Design review of the part built by this model. Coordinates are the model's own, in mm. Give positions to 0.01 mm unless a question says otherwise; leave off trailing zeros. Write each loop counter-clockwise with the first axis right and the second up, starting at its lowest first coordinate (ties: lowest second). Pieces come first, ordered by that corner, then holes. Notation, with made-up numbers: M -23,-39 L 12,-39 A6 cw 12,-34 Z; hole C 37.25,-20.75 d4. An arc over 180 degrees is marked long. Answer in a Markdown table with one row per item.
```python
from build123d import *

# Parameters (mm, degrees)
SKETCH1_W               = 105
SKETCH1_H               = 192.3454
BOSS_EXTRUDE1_DEPTH     = 3.175
CHAMFER1_SIZE           = 3.5
SKETCH2_R               = 25
CUT_EXTRUDE1_DEPTH      = 110.615322151
CUT_EXTRUDE_THIN1_START = -1
CUT_EXTRUDE_THIN1_DEPTH = 1
CUT_EXTRUDE2_DEPTH      = 1
SKETCH6_R               = 1.1
CUT_EXTRUDE3_DEPTH      = 110.615322151
CHAMFER2_SIZE           = 1.1


# Read off the part's stored shape, not the designer's step: Cut-Extrude-Thin1
with BuildPart() as part:
    # Sketch1 → Boss-Extrude1 (new body)
    with BuildSketch(Plane(origin=(0, 0, 0), x_dir=(1, 0, 0), z_dir=(0, 1, 0))):
        Rectangle(SKETCH1_W, SKETCH1_H)
    extrude(amount=BOSS_EXTRUDE1_DEPTH)

    # Chamfer1
    chamfer1_edges = [part.edges().sort_by_distance(p)[0] for p in [
        (-52.5, 1.5875, -96.1727),
        (52.5, 1.5875, -96.1727),
        (52.5, 1.5875, 96.1727),
        (-52.5, 1.5875, 96.1727),
    ]]
    chamfer(chamfer1_edges, length=CHAMFER1_SIZE)

    # Sketch2 → Cut-Extrude1 (cut, through all)
    with BuildSketch(Plane.XZ):
        with Locations(Location((0, -32.057566667, 0), (0, 0, 270))):
            Circle(SKETCH2_R)
    extrude(amount=-CUT_EXTRUDE1_DEPTH, mode=Mode.SUBTRACT)

    # Cut-Extrude-Thin1 outline → Cut-Extrude-Thin1 (cut)
    # profile 1 of 2: a face of its own
    with BuildSketch(Plane(origin=(0, 0, 0), x_dir=(-1, 0, 0), z_dir=(0, -1, 0)).offset(CUT_EXTRUDE_THIN1_START)):
        with BuildLine():
            Line((-0.5, 7.062567167), (-0.5, -10.4787141))
            ThreePointArc((-0.5, -10.4787141), (-6.237149669, -19.303333464), (-7.980739941, -29.683539926))
            ThreePointArc((-7.980739941, -29.683539926), (0, -26.804235846), (7.980739941, -29.683539926))
            ThreePointArc((7.980739941, -29.683539926), (6.237149669, -19.303333464), (0.5, -10.4787141))
            Line((0.5, -10.4787141), (0.5, 7.062567167))
            ThreePointArc((0.5, 7.062567167), (0, 7.057566667), (-0.5, 7.062567167))
        make_face()
        with BuildLine():
            ThreePointArc((0, -11.397130906), (5.003923805, -18.927747814), (6.982377972, -27.750171719))
            ThreePointArc((6.982377972, -27.750171719), (0, -25.804235846), (-6.982377972, -27.750171719))
            ThreePointArc((-6.982377972, -27.750171719), (-5.003923805, -18.927747814), (0, -11.397130906))
        make_face(mode=Mode.SUBTRACT)
    # profile 2 of 2: a face of its own
    with BuildSketch(Plane(origin=(0, 0, 0), x_dir=(-1, 0, 0), z_dir=(0, -1, 0)).offset(CUT_EXTRUDE_THIN1_START)):
        with BuildLine():
            ThreePointArc((-3.461538462, -73.83767702), (-2.032623324, -72.965633547), (-0.5, -72.292340123))
            Line((-0.5, -72.292340123), (-0.5, -96.1727))
            Line((-0.5, -96.1727), (0.5, -96.1727))
            Line((0.5, -96.1727), (0.5, -89.050988889))
            Line((0.5, -89.050988889), (5.5, -89.050988889))
            Line((5.5, -89.050988889), (5.5, -88.050988889))
            Line((5.5, -88.050988889), (0.5, -88.050988889))
            Line((0.5, -88.050988889), (0.5, -71.977550364))
            ThreePointArc((0.5, -71.977550364), (3.75, -71.547658069), (7, -71.977550364))
            Line((7, -71.977550364), (7, -96.1727))
            Line((7, -96.1727), (8, -96.1727))
            Line((8, -96.1727), (8, -81.550988889))
            Line((8, -81.550988889), (32.5, -81.550988889))
            Line((32.5, -81.550988889), (32.5, 13.3273))
            Line((32.5, 13.3273), (39, 13.3273))
            Line((39, 13.3273), (39, -88.050988889))
            Line((39, -88.050988889), (9.5, -88.050988889))
            Line((9.5, -88.050988889), (9.5, -89.050988889))
            Line((9.5, -89.050988889), (40, -89.050988889))
            Line((40, -89.050988889), (40, 13.3273))
            Line((40, 13.3273), (43.75, 13.3273))
            Line((43.75, 13.3273), (43.75, 24.3273))
            ThreePointArc((43.75, 24.3273), (41.580951895, 29.804525575), (36.25, 32.311659711))
            Line((36.25, 32.311659711), (36.25, 63.444142327))
            Line((36.25, 63.444142327), (4.25, 63.444142327))
            Line((4.25, 63.444142327), (4.25, 68.752070988))
            ThreePointArc((4.25, 68.752070988), (6.207809813, 67.846319731), (7.980739941, 66.617448963))
            ThreePointArc((7.980739941, 66.617448963), (6.237149669, 76.997655425), (0.5, 85.822274789))
            Line((0.5, 85.822274789), (0.5, 96.1727))
            Line((0.5, 96.1727), (-0.5, 96.1727))
            Line((-0.5, 96.1727), (-0.5, 85.822274789))
            ThreePointArc((-0.5, 85.822274789), (-6.237149669, 76.997655425), (-7.980739941, 66.617448963))
            ThreePointArc((-7.980739941, 66.617448963), (-6.207809813, 67.846319731), (-4.25, 68.752070988))
            Line((-4.25, 68.752070988), (-4.25, 63.444142327))
            Line((-4.25, 63.444142327), (-36.25, 63.444142327))
            Line((-36.25, 63.444142327), (-36.25, 32.311659711))
            ThreePointArc((-36.25, 32.311659711), (-41.580951895, 29.804525575), (-43.75, 24.3273))
            Line((-43.75, 24.3273), (-43.75, 13.3273))
            Line((-43.75, 13.3273), (-40, 13.3273))
            Line((-40, 13.3273), (-40, -96.1727))
            Line((-40, -96.1727), (-39, -96.1727))
            Line((-39, -96.1727), (-39, -38.185855556))
            Line((-39, -38.185855556), (-3.25, -38.185855556))
            Line((-3.25, -38.185855556), (-3.25, -29.234128142))
            ThreePointArc((-3.25, -29.234128142), (0, -28.804235846), (3.25, -29.234128142))
            Line((3.25, -29.234128142), (3.25, -44.685855556))
            Line((3.25, -44.685855556), (-31.5, -44.685855556))
            Line((-31.5, -44.685855556), (-31.5, -39.685855556))
            Line((-31.5, -39.685855556), (-32.5, -39.685855556))
            Line((-32.5, -39.685855556), (-32.5, -45.685855556))
            Line((-32.5, -45.685855556), (3.25, -45.685855556))
            Line((3.25, -45.685855556), (3.25, -53.222136322))
            ThreePointArc((3.25, -53.222136322), (-2.487149669, -62.046755686), (-4.230739941, -72.426962148))
            ThreePointArc((-4.230739941, -72.426962148), (3.75, -69.547658069), (11.730739941, -72.426962148))
            ThreePointArc((11.730739941, -72.426962148), (9.987149669, -62.046755686), (4.25, -53.222136322))
            Line((4.25, -53.222136322), (4.25, -29.548917901))
            ThreePointArc((4.25, -29.548917901), (5.782623324, -30.222211325), (7.211538462, -31.094254798))
            Line((7.211538462, -31.094254798), (7.788461538, -30.277456314))
            ThreePointArc((7.788461538, -30.277456314), (0, -27.804235846), (-7.788461538, -30.277456314))
            Line((-7.788461538, -30.277456314), (-7.211538462, -31.094254798))
            ThreePointArc((-7.211538462, -31.094254798), (-5.782623324, -30.222211325), (-4.25, -29.548917901))
            Line((-4.25, -29.548917901), (-4.25, -37.185855556))
            Line((-4.25, -37.185855556), (-39, -37.185855556))
            Line((-39, -37.185855556), (-39, 13.3273))
            Line((-39, 13.3273), (-32.5, 13.3273))
            Line((-32.5, 13.3273), (-32.5, -35.685855556))
            Line((-32.5, -35.685855556), (-31.5, -35.685855556))
            Line((-31.5, -35.685855556), (-31.5, 13.3273))
            Line((-31.5, 13.3273), (-27.75, 13.3273))
            Line((-27.75, 13.3273), (-27.75, 24.3273))
            ThreePointArc((-27.75, 24.3273), (-29.919048105, 29.804525575), (-35.25, 32.311659711))
            Line((-35.25, 32.311659711), (-35.25, 62.444142327))
            Line((-35.25, 62.444142327), (-3.25, 62.444142327))
            Line((-3.25, 62.444142327), (-3.25, 69.066860747))
            ThreePointArc((-3.25, 69.066860747), (0, 69.496753043), (3.25, 69.066860747))
            Line((3.25, 69.066860747), (3.25, 62.444142327))
            Line((3.25, 62.444142327), (35.25, 62.444142327))
            Line((35.25, 62.444142327), (35.25, 32.311659711))
            ThreePointArc((35.25, 32.311659711), (29.919048105, 29.804525575), (27.75, 24.3273))
            Line((27.75, 24.3273), (27.75, 13.3273))
            Line((27.75, 13.3273), (31.5, 13.3273))
            Line((31.5, 13.3273), (31.5, -80.550988889))
            Line((31.5, -80.550988889), (8, -80.550988889))
            Line((8, -80.550988889), (8, -72.292340123))
            ThreePointArc((8, -72.292340123), (9.532623324, -72.965633547), (10.961538462, -73.83767702))
            Line((10.961538462, -73.83767702), (11.538461538, -73.020878536))
            ThreePointArc((11.538461538, -73.020878536), (3.75, -70.547658069), (-4.038461538, -73.020878536))
            Line((-4.038461538, -73.020878536), (-3.461538462, -73.83767702))
        make_face()
        with BuildLine():
            ThreePointArc((3.75, -54.140553128), (8.753923805, -61.671170036), (10.732377972, -70.493593942))
            ThreePointArc((10.732377972, -70.493593942), (3.75, -68.547658069), (-3.232377972, -70.493593942))
            ThreePointArc((-3.232377972, -70.493593942), (-1.253923805, -61.671170036), (3.75, -54.140553128))
        make_face(mode=Mode.SUBTRACT)
        with BuildLine():
            Line((-28.75, 14.3273), (-42.75, 14.3273))
            Line((-42.75, 14.3273), (-42.75, 24.3273))
            ThreePointArc((-42.75, 24.3273), (-35.75, 31.3273), (-28.75, 24.3273))
            Line((-28.75, 24.3273), (-28.75, 14.3273))
        make_face(mode=Mode.SUBTRACT)
        with BuildLine():
            ThreePointArc((28.75, 24.3273), (35.75, 31.3273), (42.75, 24.3273))
            Line((42.75, 24.3273), (42.75, 14.3273))
            Line((42.75, 14.3273), (28.75, 14.3273))
            Line((28.75, 14.3273), (28.75, 24.3273))
        make_face(mode=Mode.SUBTRACT)
        with BuildLine():
            ThreePointArc((0, 84.903857983), (5.003923805, 77.373241075), (6.982377972, 68.55081717))
            ThreePointArc((6.982377972, 68.55081717), (0, 70.496753043), (-6.982377972, 68.55081717))
            ThreePointArc((-6.982377972, 68.55081717), (-5.003923805, 77.373241075), (0, 84.903857983))
        make_face(mode=Mode.SUBTRACT)
    extrude(amount=CUT_EXTRUDE_THIN1_DEPTH, mode=Mode.SUBTRACT)

    # Sketch4 → Cut-Extrude2 (cut)
    with BuildSketch(Plane.XZ):
        with BuildLine():
            Line((-10.5, 88.050988889), (-9.5, 88.050988889))
            ThreePointArc((-9.5, 88.050988889), (-7.5, 86.050988889), (-5.5, 88.050988889))
            Line((-5.5, 88.050988889), (-4.5, 88.050988889))
            ThreePointArc((-4.5, 88.050988889), (-7.5, 85.050988889), (-10.5, 88.050988889))
        make_face()
        with BuildLine():
            Line((31.5, 35.685855556), (31.5, 34.685855556))
            ThreePointArc((31.5, 34.685855556), (28.5, 37.685855556), (31.5, 40.685855556))
            Line((31.5, 40.685855556), (31.5, 39.685855556))
            ThreePointArc((31.5, 39.685855556), (29.5, 37.685855556), (31.5, 35.685855556))
        make_face()
    extrude(amount=-CUT_EXTRUDE2_DEPTH, mode=Mode.SUBTRACT)

    # Sketch6 → Cut-Extrude3 (cut, through all)
    with BuildSketch(Plane.XZ):
        with Locations(Location((48.628679656, -20.801379656, 0), (0, 0, 270))):
            Circle(SKETCH6_R)
        with Locations(Location((-48.628679656, 92.301379656, 0), (0, 0, 270))):
            Circle(SKETCH6_R)
        with Locations(Location((-48.628679656, 35.75, 0), (0, 0, 270))):
            Circle(SKETCH6_R)
        with Locations(Location((-48.628679656, -20.801379656, 0), (0, 0, 270))):
            Circle(SKETCH6_R)
        with Locations(Location((-48.628679656, -92.301379656, 0), (0, 0, 270))):
            Circle(SKETCH6_R)
        with Locations(Location((48.628679656, -92.301379656, 0), (0, 0, 270))):
            Circle(SKETCH6_R)
        with Locations(Location((48.628679656, 35.75, 0), (0, 0, 270))):
            Circle(SKETCH6_R)
        with Locations(Location((48.628679656, 92.301379656, 0), (0, 0, 270))):
            Circle(SKETCH6_R)
    extrude(amount=-CUT_EXTRUDE3_DEPTH, mode=Mode.SUBTRACT)

    # Chamfer2
    chamfer2_edges = [part.edges().sort_by_distance(p)[0] for p in [
        (48.628679656, 0, 93.401379656),
        (48.628679656, 0, 36.85),
        (48.628679656, 0, -91.201379656),
        (-48.628679656, 0, -91.201379656),
        (-48.628679656, 0, -19.701379656),
        (-48.628679656, 0, 36.85),
        (-48.628679656, 0, 93.401379656),
        (48.628679656, 0, -19.701379656),
    ]]
    chamfer(chamfer2_edges, length=CHAMFER2_SIZE)


solid = part.part
```
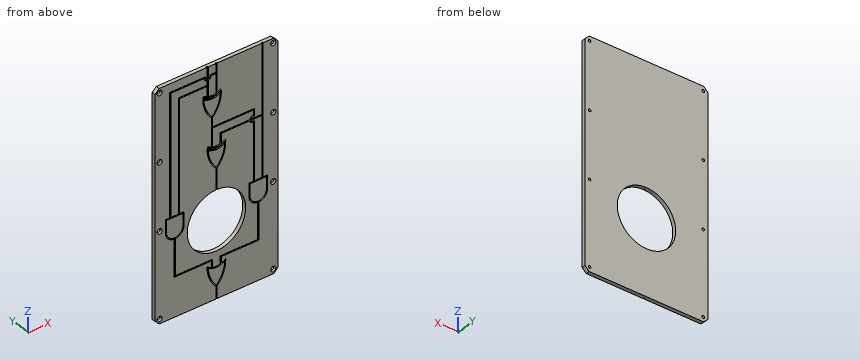
1) Add section A-A (x = 22). Write out the cut boundary in (y, z) (3 decimals).
Geometry says:
| item | result |
|---|---|
| outline | M 0,-96.173 L 3.175,-96.173 L 3.175,-43.932 L 0,-43.932 L 0,-62.444 L 1,-62.444 L 1,-63.444 L 0,-63.444 Z; M 0,-20.183 L 3.175,-20.183 L 3.175,96.173 L 0,96.173 L 0,45.686 L 1,45.686 L 1,44.686 L 0,44.686 L 0,38.186 L 1,38.186 L 1,37.186 L 0,37.186 Z |
2) To check wall thickness, follow probe 1 along X at (y, z) = (0.85, 82.5); probe 2 along Z at (x, y) = (19, 0.9); probe 3 along X at (y, z) = (0.8, 63). State the ranges of each line that lie inside material, in increasing order. Write a range as [from, to].
Geometry says:
| item | result |
|---|---|
| probe 1 | [-52.5, -40], [-39, -8], [-7, -0.5], [0.5, 39], [40, 52.5] |
| probe 2 | [-96.17, -63.44], [-62.44, -48.31], [-15.81, 37.19], [38.19, 44.69], [45.69, 96.17] |
| probe 3 | [-52.5, -40], [-39, -32.5], [-31.5, -10.34], [-9.28, 1.78], [2.84, 39], [40, 52.5] |
3) Insertion check: P1, Ø3, axis at x = 21, z = 59, coming from the -Y side. The pin has a flat end and moves straight along its axis. Give the tip position at first contact, or say it passes through.
Geometry says:
| item | result |
|---|---|
| P1 | y = 0 |
4) Add section C-C (z = -44.5). Write out the cut boundary in (x, y) (3 decimals), and give its area (3 significant figures).
Geometry says:
| item | result |
|---|---|
| outline | M -52.5,0 L -36.25,0 L -36.25,1 L -35.25,1 L -35.25,0 L -21.684,0 L -21.684,3.175 L -52.5,3.175 Z; M 21.684,0 L 35.25,0 L 35.25,1 L 36.25,1 L 36.25,0 L 52.5,0 L 52.5,3.175 L 21.684,3.175 Z |
| area | 194 mm^2 |
5) Add section B-B (y = 2.25). Count the separate pieces of the cut face and the enclosed holes in it, and give its area (3 significant figures).
Geometry says:
| item | result |
|---|---|
| separate pieces | 1 |
| enclosed holes | 9 |
| area | 18,200 mm^2 |
